Autodesk Inventor part; units mm, degrees
ref_plane "YZ Plane" through (0, 0, 0) normal (1, 0, 0) x (0, 1, 0)
ref_plane "XZ Plane" through (0, 0, 0) normal (0, 1, 0) x (-1, 0, 0)
ref_plane "XY Plane" through (0, 0, 0) normal (0, 0, 1) x (1, 0, 0)
sketch "Sketch1" plane through (0, 0, 0) normal (0, 0, 1) x (1, 0, 0)
  line L0 (-50.5, 47.5) -> (50.5, 47.5)
  line L1 (50.5, 47.5) -> (50.5, -47.5)
  line L2 (50.5, -47.5) -> (-50.5, -47.5)
  line L3 (-50.5, -47.5) -> (-50.5, 47.5)
  point P0 (0, 0)
  point P1 (0, 47.5)
  point P2 (-50.5, 0)
  dimension "d0" = 95
  dimension "d1" = 101
extrude "Extrusion1" add sketch "Sketch1" along normal blind 20
sketch "Sketch2" plane through (0, 0, 20) normal (0, 0, 1) x (1, 0, 0)
  line L0 (-50.5, 47.5) -> (-50.5, -47.5)
  line L1 (-50.5, -47.5) -> (50.5, -47.5)
  line L2 (50.5, -47.5) -> (50.5, 47.5)
  line L3 (50.5, 47.5) -> (-50.5, 47.5)
  line L4 (-47.5, 44.5) -> (-47.5, -44.5)
  line L5 (-47.5, -44.5) -> (47.5, -44.5)
  line L6 (47.5, -44.5) -> (47.5, 44.5)
  line L7 (47.5, 44.5) -> (-47.5, 44.5)
  point P0 (0, 0)
  dimension "d4" = 3
extrude "Extrusion2" cut sketch "Sketch2" against normal blind 15 contours L7 L6 L5 L4
sketch "Sketch3" plane through (0, 0, 5) normal (0, 0, 1) x (1, 0, 0)
  line L0 (-25.5, 37) -> (-5.5, 37)
  line L1 (-25.5, 28) -> (-25.5, 37)
  line L2 (-5.5, 28) -> (-25.5, 28)
  line L3 (-5.5, 37) -> (-5.5, 28)
  line L4 (4.5, 37) -> (24.5, 37)
  line L5 (4.5, 28) -> (4.5, 37)
  line L6 (24.5, 28) -> (4.5, 28)
  line L7 (24.5, 37) -> (24.5, 28)
  line L8 (-4.5, 38) -> (-26.5, 38)
  line L9 (-26.5, 38) -> (-26.5, 27)
  line L10 (-26.5, 27) -> (-4.5, 27)
  line L11 (-4.5, 27) -> (-4.5, 38)
  line L12 (25.5, 38) -> (3.5, 38)
  line L13 (3.5, 38) -> (3.5, 27)
  line L14 (3.5, 27) -> (25.5, 27)
  line L15 (25.5, 27) -> (25.5, 38)
  point P0 (0, 0)
  dimension "d7" = 1
  dimension "d8" = 1
extrude "Extrusion3" cut sketch "Sketch3" against normal through all contours L0 L3 L2 L1 | L4 L7 L6 L5 | L11 L10 L9 L8 | L15 L14 L13 L12
sketch "Sketch4" plane through (0, 0, 5) normal (0, 0, 1) x (1, 0, 0)
  circle A0 centre (-44, -24) radius 1.5
  circle A1 centre (44, -24) radius 1.5
  circle A2 centre (44, 41) radius 1.5
  circle A3 centre (-44, 41) radius 1.5
  circle A4 centre (-44, -24) radius 5
  circle A5 centre (44, -24) radius 5
  circle A6 centre (-44, 41) radius 5
  circle A7 centre (44, 41) radius 5
  point P0 (0, 0)
  dimension "d11" = 10
  dimension "d12" = 10
  dimension "d13" = 10
  dimension "d14" = 10
extrude "Extrusion4" add sketch "Sketch4" along normal blind 9.5
fillet "Fillet1" radius 10 8 edges at (-47.5, -27.5707, 9.75) (-47.5, -20.4293, 9.75) (47.5, -20.4293, 9.75) (47.5, -27.5707, 9.75) (47.5, 37.4293, 9.75) (40.4293, 44.5, 9.75) (-40.4293, 44.5, 9.75) (-47.5, 37.4293, 9.75)
sketch "Sketch7" plane through (-50.5, -47.5, 0) normal (-1, 0, 0) x (0, 0, 1)
  line L0 (10, 73.75) -> (16, 73.75)
  line L1 (16, 73.75) -> (16, 38.75)
  line L2 (16, 38.75) -> (10, 38.75)
  line L3 (10, 38.75) -> (10, 73.75)
  line L4 (20, 95) -> (20, 0)
  line L5 (0, 0) -> (20, 0)
  point P0 (0, 47.5)
  dimension "d18" = 6
  dimension "d19" = 35
  dimension "d20" = 4
  dimension "d21" = 38.75
extrude "Extrusion5" cut sketch "Sketch7" against normal up to surface (3 mm away)
sketch "Sketch9" plane through (0, 0, 5) normal (0, 0, 1) x (1, 0, 0)
  circle A0 centre (0, -1.5) radius 2.5 construction
  circle A1 centre (0, -37.5) radius 2.5 construction
  point P0 (0, 0)
hole "Hole2" at (0, -1.5, 5) at (0, -37.5, 5) direction (0, 0, -1) diameter 4 end through all countersink diameter 8 countersink angle 90
properties part number "10-06-004 carcasa spate"
Here's how the part is built. I have some questions about the finished solid (model axes, mm). A direction names the side the tool comes from. Give positions to 0.01 mm unless a question says otherwise; leave off trailing zeros. Loops run counter-clockwise (first coordinate to the right, second up) from the corner with the lowest first, then second, coordinate; pieces in that order, holes last. Notation, with made-up numbers: (34.5, -18) -> (90.5, -18) arc R16 cw to (90.5, 0) -> close; hole circle Ø5 at (51, -25). An arc over 180 degrees is marked (long way). Answer as a JSON object with one key per item and string values. Group by question number.
Item 1: Imagine slicing it at D-D on z = 12. Give the number of separate pieces and of enclosed holes in the cut face, then the cut area to 3 significant figures.
Item 2: Imagine slicing it at A-A on z = 18.75. Write out the boundary of the cut face in (x, y).
Item 3: Will these pins go through, and if not, where does the flat tip stop? pin 1 (3 mm diameter, centred on x = 0, y = -37.5, fed in from -Z); pin 2 (3.5 mm diameter, centred on x = -44, y = 41, fed in from +Z); pin 3 (1.5 mm diameter, centred on x = -26, y = 1.5, fed in from +Z).
Item 4: I need wall thicknesses on L1, parallel to Y at x = 0, z = 0.75; L2, parallel to Y at x = -19.5, z = 15.5; L3, parallel to X at y = -1.5, z = 1.15. Which ranges of each line are inside material? Lowest first, please.
Item 5: On a 3-axis mill with a long thin cutter (end or side, diameter ignored), from which of +Z, -Z, +X, -X, +Y, -Y can I reach the whole of each face in a straight line? I mean faces 5 (the flat face through (-4.5, 32, 3)), 6 (the flat face through (-4, -46, 20)), 7 (the cylindrical face through (-45.2, 41.9, 9.7)). Say none if no direction works.
Item 6: Imagine slicing it at C-C on y = 16. Write out the boundary of the cut face in (x, z), then the cut area to 3 significant figures.
Item 7: Thinking about a two-plate mould opening in X: for faces 1 (the flat face through (3.5, 33, 3)), 2 (the cylindrical face through (45.924, 32.871, 9.683)), 3 (the flat face through (-49, 26.25, 13)), 4 (the flat face through (50.5, 1, 10)), which applies, pulls with the +X half, pulls with the -X half, needs draft (parallel to the pull), parting line crosses it, or undercut?
Item 8: Imagine slicing it at B-B on x = 18.5. Write out the boundary of the cut face in (y, z).
Answer list:
{
 "1": {"separate pieces": "1", "enclosed holes": "4", "area": "1,390 mm2"},
 "2": {"outline": "(-50.5, -47.5) -> (50.5, -47.5) -> (50.5, 47.5) -> (-50.5, 47.5) -> close; hole (-47.5, -44.5) -> (47.5, -44.5) -> (47.5, 44.5) -> (-47.5, 44.5) -> close"},
 "3": {"pin 1": "passes through", "pin 2": "stops at z = 14.5", "pin 3": "stops at z = 5"},
 "4": {"L1": "y = -47.5 to -39.5, -35.5 to -3.5, 0.5 to 47.5", "L2": "y = -47.5 to -44.5, 44.5 to 47.5", "L3": "x = -50.5 to -2, 2 to 50.5"},
 "5": {"face 5": "+Z, -Z", "face 6": "+Z, +X, -X, +Y, -Y", "face 7": "+Z"},
 "6": {"outline": "(-50.5, 0) -> (50.5, 0) -> (50.5, 20) -> (47.5, 20) -> (47.5, 5) -> (-47.5, 5) -> (-47.5, 10) -> (-50.5, 10) -> close; (-50.5, 16) -> (-47.5, 16) -> (-47.5, 20) -> (-50.5, 20) -> close", "area": "577 mm2"},
 "7": {"face 1": "undercut", "face 2": "undercut", "face 3": "needs draft", "face 4": "pulls with the +X half"},
 "8": {"outline": "(-47.5, 0) -> (27, 0) -> (27, 5) -> (-44.5, 5) -> (-44.5, 20) -> (-47.5, 20) -> close; (38, 0) -> (47.5, 0) -> (47.5, 20) -> (44.5, 20) -> (44.5, 5) -> (38, 5) -> close"}
}
